Read the model definition and answer for the solid it produces. Units are mm, in the model's axes. Face numbers are marked on the shaded views. Give positions to 0.01 mm unless a question says otherwise; leave off trailing zeros. Loops run counter-clockwise (first coordinate to the right, second up) from the corner with the lowest first, then second, coordinate; pieces in that order, holes last. Notation, with made-up numbers: (-26, 75) -> (22, 75) arc R17 ccw to (22, 103) -> close; hole circle Ø7 at (-3.75, 12.25). An arc over 180 degrees is marked (long way). Return JSON: item names as keys, results as strings. Group by question number.
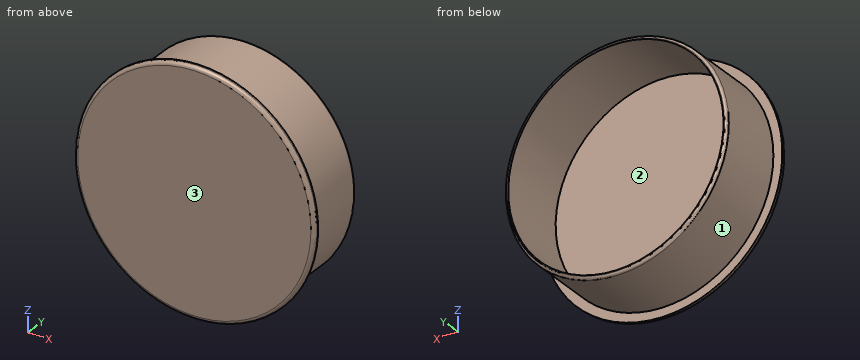
from build123d import *

# Parameters (mm, degrees)
SKETCH1_R           = 62
BOSS_EXTRUDE1_DEPTH = 42
SKETCH2_R           = 67
BOSS_EXTRUDE2_DEPTH = 3
FILLET1_R           = 2
SHELL1_T            = -2
FILLET2_R           = 1.4


with BuildPart() as part:
    # Sketch1 → Boss-Extrude1 (new body)
    with BuildSketch(Plane(origin=(0, 0, 0), x_dir=(1, 0, 0), z_dir=(0, 1, 0))):
        with Locations(Location((0, 0, 0), (0, 0, 90))):
            Circle(SKETCH1_R)
    extrude(amount=BOSS_EXTRUDE1_DEPTH)

    # Sketch2 → Boss-Extrude2 (add)
    with BuildSketch(Plane(origin=(0, 0, 0), x_dir=(1, 0, 0), z_dir=(0, 1, 0))):
        with Locations(Location((0, 0, 0), (0, 0, 270))):
            Circle(SKETCH2_R)
    extrude(amount=BOSS_EXTRUDE2_DEPTH)

    # Fillet1
    fillet1_edges = [part.edges().sort_by_distance(p)[0] for p in [
        (0, 0, -67),
    ]]
    fillet(fillet1_edges, radius=FILLET1_R)

    # Shell1
    shell1_openings = [part.faces().sort_by_distance(p)[0] for p in [
        (0, 42, 0),
    ]]
    offset(amount=SHELL1_T, openings=shell1_openings, kind=Kind.INTERSECTION)

    # Fillet2
    fillet2_edges = [part.edges().sort_by_distance(p)[0] for p in [
        (0, 42, 62),
    ]]
    fillet(fillet2_edges, radius=FILLET2_R)


solid = part.part
1. Section C-C on y = 6 is taken. Determine the outline of the cut face in (x, z).
2. Section A-A on x = 0 is taken. Determine the outline of the cut face in (y, z), then the cut area to 3 significant figures.
3. Flat-ended cylindrical pins translate along their axes: pin 1 Ø4 at (x, y) = (-2.5, 11.5) entering from -Z; pin 2 Ø6 at (x, y) = (32.5, 5.5) entering from -Z; pin 3 Ø5 at (x, y) = (8, 30.5) entering from +Z. Find the tip coordinate at first contact, or state that the pin passes through.
4. Determine the mould class of the marked faces 1, 2 and 3 for opening direction X: pulls with the +X half, pulls with the -X half, needs draft (parallel to the pull), parting line crosses it, or undercut.
5. Section B-B on z = 0 is taken. Determine the outline of the cut face in (x, y), then the cut area to 3 significant figures.
6. Straight lines are drawn through the part: line 1 (X direction, y = 9, z = 2); line 2 (Y direction, x = -11, z = -36); line 3 (Z direction, x = -12, y = 24.5). For each, find the intervals that lie inside material, in ascending order. Write a range as from..to.
Completed:
{
 "1": {"outline": "circle Ø124 at (0, 0); hole circle Ø120 at (0, 0)"},
 "2": {"outline": "(0, -65) arc R2 ccw to (2, -67) -> (3, -67) -> (3, -62) -> (40.6, -62) arc R1.4 ccw to (42, -60.6) -> (42, -60) -> (2, -60) -> (2, 60) -> (42, 60) -> (42, 60.6) arc R1.4 ccw to (40.6, 62) -> (3, 62) -> (3, 67) -> (2, 67) arc R2 ccw to (0, 65) -> close", "area": "435 mm²"},
 "3": {"pin 1": "stops at z = -62", "pin 2": "stops at z = -59.48", "pin 3": "stops at z = 61.76"},
 "4": {"face 1": "parting line crosses it", "face 2": "undercut", "face 3": "needs draft"},
 "5": {"outline": "(-67, 2) arc R2 ccw to (-65, 0) -> (65, 0) arc R2 ccw to (67, 2) -> (67, 3) -> (62, 3) -> (62, 40.6) arc R1.4 ccw to (60.6, 42) -> (60, 42) -> (60, 2) -> (-60, 2) -> (-60, 42) -> (-60.6, 42) arc R1.4 ccw to (-62, 40.6) -> (-62, 3) -> (-67, 3) -> close", "area": "435 mm²"},
 "6": {"line 1": "x = -61.97..-59.97, 59.97..61.97", "line 2": "y = 0..2", "line 3": "z = -60.83..-58.79, 58.79..60.83"}
}
